Autodesk Inventor part; units mm, degrees
ref_plane "YZ Plane" through (0, 0, 0) normal (1, 0, 0) x (0, 1, 0)
ref_plane "XZ Plane" through (0, 0, 0) normal (0, 1, 0) x (-1, 0, 0)
ref_plane "XY Plane" through (0, 0, 0) normal (0, 0, 1) x (1, 0, 0)
sketch "Sketch1" plane through (0, 0, 0) normal (0, 1, 0) x (-1, 0, 0)
  line L0 (82, 0) -> (82, -52)
  line L1 (82, -52) -> (0, -52)
  line L2 (0, -52) -> (0, 0)
  line L3 (82, 0) -> (0, 0)
  line L4 (0, 0) -> (76.656, -52)
  line L5 (82, -52) -> (5.344, 0)
  line L6 (82, -26) -> (0, -26) construction
  line L7 (0, -52) -> (76.656, 0)
  line L8 (82, 0) -> (5.344, -52)
  line L9 (41, -52) -> (41, 0) construction
  line L10 (82, -49) -> (0, -49)
  line L11 (3, -52) -> (3, -32)
  line L12 (3, -32) -> (0, -32)
  line L13 (79, -52) -> (79, -32)
  line L14 (79, -32) -> (82, -32)
  line L15 (76.656, 0) -> (76.656, 1.5)
  line L16 (76.656, 1.5) -> (82, 1.5)
  line L17 (82, 1.5) -> (82, 0)
  line L18 (5.344, 0) -> (5.344, 1.5)
  line L19 (5.344, 1.5) -> (0, 1.5)
  line L20 (0, 1.5) -> (0, 0)
  point P0 (43.672, -26)
  point P1 (41, -24.1874)
  point P2 (38.328, -26)
  point P3 (4.4225, -49)
  point P4 (0, -49)
  point P5 (77.5775, -49)
  point P6 (41, -27.8126)
  point P7 (72.2336, -49)
  point P8 (9.7664, -49)
  point P9 (79, -49)
  point P10 (3, -49)
  dimension "d5" = 82
  dimension "d6" = 52
  dimension "d7" = 3
  dimension "d9" = 3
  dimension "d12" = 20
  dimension "d13" = 3
  dimension "d14" = 20
  dimension "d15" = 3
  dimension "d35" = 1.5
extrude "Extrusion1" add sketch "Sketch1" along normal blind 3 contours L8 L5 L7 L3 | L3 L15 L16 L17 | L0 L10 L13 L14 | L8 L4 L7 L5 | L5 L10 L4 L8 | L0 L5 L13 L10 | L5 L7 L4 L3 | L3 L20 L19 L18 | L10 L13 L5 | L5 L13 L1 L4 L10 | L8 L10 L7 L4 | L1 L13 L5 | L4 L1 L8 L10 | L8 L1 L11 L7 L10 | L12 L11 L10 L2 | L7 L11 L10 | L10 L11 L7 L2 | L11 L1 L7
sketch "Sketch2" plane through (0, 0, -52) normal (0, 0, -1) x (-1, 0, 0)
  line L0 (0, 3) -> (38.328, 3)
  line L1 (82, 0) -> (76.656, 0)
  line L2 (0, 3) -> (82, 3)
  line L3 (82, 3) -> (82, 0)
  line L4 (82, 0) -> (0, 0)
  line L5 (0, 0) -> (0, 3)
  line L6 (0, 3) -> (0, 10.5)
  line L7 (0, 10.5) -> (20, 10.5)
  line L8 (20, 10.5) -> (32.9904, 3)
  line L9 (11.7, 9.2) -> (15.9, 9.2)
  line L10 (15.9, 9.2) -> (15.9, 4)
  line L11 (15.9, 4) -> (11.7, 4)
  line L12 (11.7, 4) -> (11.7, 9.2)
  line L13 (41, 0) -> (41, 19.2831) construction
  line L14 (32.9904, 3) -> (41, 3) construction
  line L15 (82, 3) -> (43.672, 3)
  line L16 (82, 3) -> (0, 3)
  line L17 (82, 0) -> (82, 3)
  line L18 (82, 3) -> (82, 10.5)
  line L19 (82, 10.5) -> (62, 10.5)
  line L20 (62, 10.5) -> (49.0096, 3)
  line L21 (70.3, 9.2) -> (66.1, 9.2)
  line L22 (66.1, 9.2) -> (66.1, 4)
  line L23 (66.1, 4) -> (70.3, 4)
  line L24 (70.3, 4) -> (70.3, 9.2)
  line L25 (49.0096, 3) -> (41, 3) construction
  point P0 (11.7, 6.6)
  point P1 (13.8, 4)
  point P2 (13.8, 9.2)
  point P3 (70.3, 6.6)
  point P4 (68.2, 4)
  point P5 (68.2, 9.2)
  point P6 (38.328, 3)
  dimension "d16" = 20
  dimension "d17" = 7.5
  dimension "d18" = 15
  dimension "d19" = 11.7
  dimension "d20" = 4.2
  dimension "d21" = 5.2
  dimension "d22" = 4
extrude "Extrusion2" add sketch "Sketch2" along normal blind 1.5
sketch "Sketch3" plane through (0, 0, -32) normal (1, 0, 0) x (0, 0, -1)
  line L0 (21.5, 0) -> (21.5, 10.5)
  line L1 (21.5, 10.5) -> (11.5, 10.5)
  line L2 (0, 0) -> (21.5, 0)
  line L3 (0, 0) -> (0, 3)
  line L4 (21.5, 0) -> (0, 0)
  line L5 (0, 0) -> (0, 3)
  line L6 (0, 3) -> (21.5, 3)
  line L7 (21.5, 3) -> (21.5, 0)
  line L8 (11.5, 10.5) -> (0, 3)
  point P0 (-32, 0)
  dimension "d25" = 10
extrude "Extrusion3" add sketch "Sketch3" along normal blind 1.5
sketch "Sketch4" plane through (-82, 0, -32) normal (-1, 0, 0) x (0, 0, 1)
  line L0 (-11.5, 10.5) -> (0, 3)
  line L1 (0, 3) -> (-11.5, 10.5)
  line L2 (-20, 10.5) -> (-21.5, 10.5)
  line L3 (-11.5, 10.5) -> (-21.5, 10.5)
  line L4 (-21.5, 10.5) -> (-21.5, 0)
  line L5 (-21.5, 0) -> (0, 0)
  line L6 (0, 0) -> (0, 3)
  line L7 (-17, 9.5) -> (-12.5, 9.5)
  line L8 (-12.5, 9.5) -> (-12.5, 4)
  line L9 (-12.5, 4) -> (-17, 4)
  line L10 (-17, 4) -> (-17, 9.5)
  point P0 (32, 0)
  point P1 (-21.5, 5.25)
  point P2 (-20, 10.5)
  dimension "d28" = 4.5
  dimension "d29" = 4.5
  dimension "d30" = 4
  dimension "d31" = 5.5
  dimension "d32" = 1
extrude "Extrusion4" add sketch "Sketch4" along normal blind 1.5
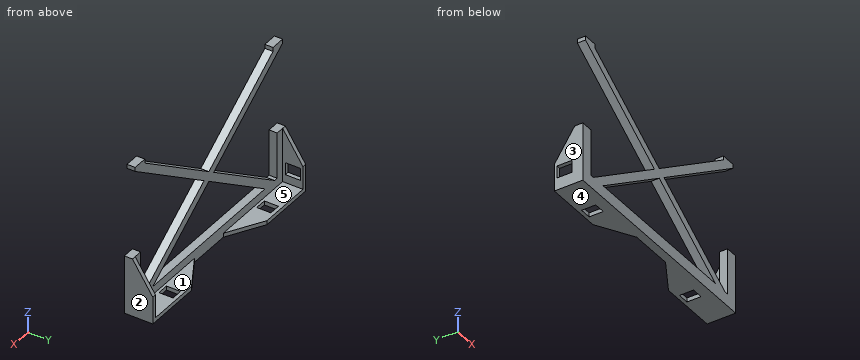
Read the model definition and answer for the solid it produces. Units are mm, in the model's axes. Face numbers are marked on the shaded views. A direction names the side the tool comes from. Round coordinates to 2 decimals unless told otherwise and drop trailing zeros. Write each loop counter-clockwise with the first axis right and the second up, starting at its lowest first coordinate (ties: lowest second). Pieces come first, ordered by that corner, then holes. Notation, with made-up numbers: (-30, 48.5) - (20, 48.5) arc R20 ccw to (20, 65.5) - close; hole circle Ø4 at (32.25, 85). An arc over 180 degrees is marked (long way). Use CSV: the item, a comma, the result in double quotes.
Q1. Each of these flat-tipped pins is pushed along its axis until it touches: pin 1 Ø1.2 at (x, z) = (-82.5, -45.5) entering from -Y; pin 2 Ø0.8 at (y, z) = (2, 0.5) entering from +X; pin 3 Ø1.6 at (y, z) = (1.5, 1) entering from -X; pin 4 Ø2 at (x, y) = (-27.5, 2) entering from +Z. Where does it stop, or does it pass through?
Values:
pin 1,"stops at y = 0"
pin 2,"stops at x = 0"
pin 3,"stops at x = -82"
pin 4,"stops at z = -14.35"
Q2. Find section B-B, the plane z = -39. Write down the section's boundary in (x, y).
Values:
outline,"(-83.5, 0) - (-79, 0) - (-79, 3) - (-82, 3) - (-82, 7.57) - (-83.5, 7.57) - close; (-62.84, 0) - (-57.49, 0) - (-57.49, 3) - (-62.84, 3) - close; (-24.51, 0) - (-19.16, 0) - (-19.16, 3) - (-24.51, 3) - close; (-3, 0) - (1.5, 0) - (1.5, 7.57) - (0, 7.57) - (0, 3) - (-3, 3) - close"
Q3. A tool of negligible diameter and unlimited length cuts with its end or side. For the marked faces 1 and 2, from which of +Z, -Z, +X, -X, +Y, -Y can it reach the whole face along a straight path? Write none if from no direction.
Values:
face 1,"+Z, +Y"
face 2,"+Z, -Z, +X, +Y, -Y"
Q4. Find section A-A, the plane x = -17. Write down the section's boundary in (y, z), then the cut area to 3 significant figures.
Values:
outline,"(0, -53.5) - (10.5, -53.5) - (10.5, -52) - (3, -52) - (3, -49) - (0, -49) - close; (0, -44.09) - (3, -44.09) - (3, -40.47) - (0, -40.47) - close; (0, -11.53) - (3, -11.53) - (3, -7.91) - (0, -7.91) - close"
area,"46.5 mm²"
Q5. Straight lines are drawn through the part: line 1 along X through (y, z) = (6.25, -39); line 2 along Z through (x, y) = (-33, 2.75); line 3 along X through (y, z) = (2.5, -44.5). For each, find the intervals that lie inside material, in ascending order.
Values:
line 1,"x = -83.5 to -82, 0 to 1.5"
line 2,"z = -53.5 to -49, -33.24 to -29.61, -22.39 to -18.76"
line 3,"x = -83.5 to -79, -70.94 to -65.6, -16.4 to -11.06, -3 to 1.5"
Q6. Determine the mould class of the marked faces 3, 4 and 5 for opening direction X: +X half, -X half, draft (parallel to the pull), parting line (faces both ways), or undercut.
Values:
face 3,"-X half"
face 4,"draft"
face 5,"undercut"
Q7. Find section D-D, the plane y = 5.75. Write down the section's boundary in (x, z), then the cut area to 3 significant figures.
Values:
outline,"(-83.5, -53.5) - (-70.3, -53.5) - (-70.3, -52) - (-82, -52) - (-82, -49) - (-83.5, -49) - close; (-83.5, -44.5) - (-82, -44.5) - (-82, -36.22) - (-83.5, -36.22) - close; (-66.1, -53.5) - (-53.77, -53.5) - (-53.77, -52) - (-66.1, -52) - close; (-28.23, -53.5) - (-15.9, -53.5) - (-15.9, -52) - (-28.23, -52) - close; (-11.7, -53.5) - (1.5, -53.5) - (1.5, -36.22) - (0, -36.22) - (0, -52) - (-11.7, -52) - close"
area,"117 mm²"
Q8. Find section C-C, the plane x = -67. Write down the section's boundary in (y, z).
Values:
outline,"(0, -53.5) - (4, -53.5) - (4, -52) - (3, -52) - (3, -49) - (0, -49) - close; (0, -45.45) - (3, -45.45) - (3, -41.82) - (0, -41.82) - close; (0, -10.18) - (3, -10.18) - (3, -6.55) - (0, -6.55) - close; (9.2, -53.5) - (10.5, -53.5) - (10.5, -52) - (9.2, -52) - close"
